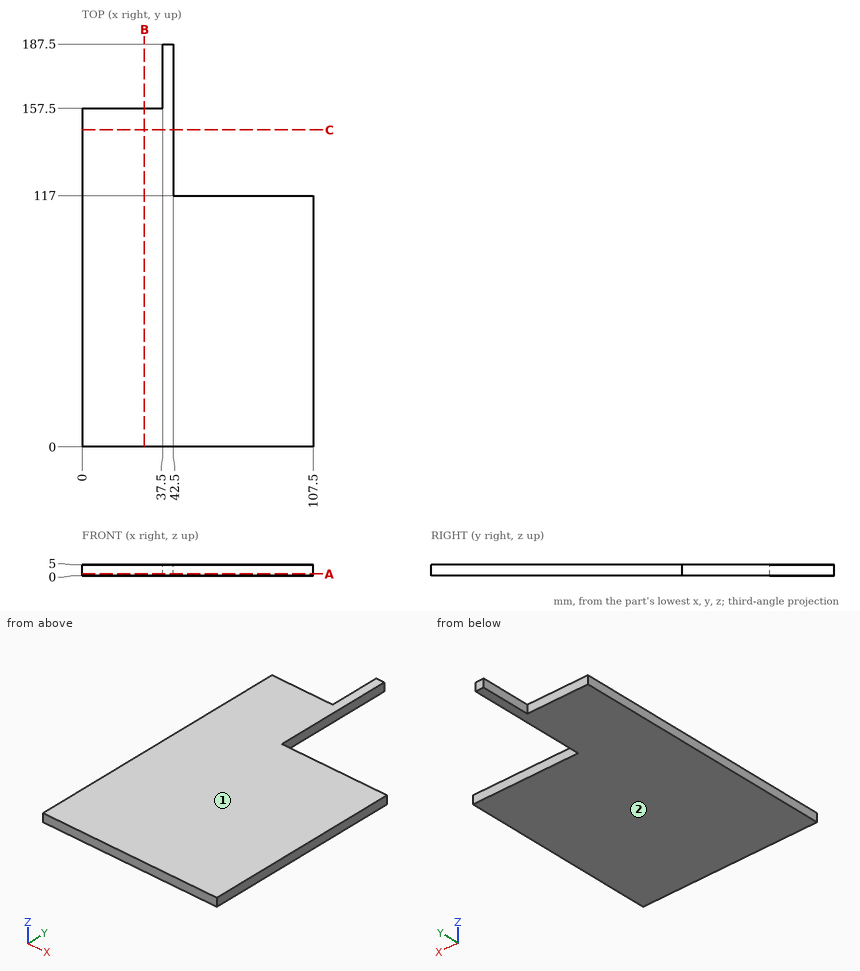
Could you check a few things on this drawing? It's one solid part, dimensions in mm from its lowest x, y, z. Coordinates: 2 decimals unless noted, no trailing zeros. Write each loop counter-clockwise with the first axis right and the second up, starting at its lowest first coordinate (ties: lowest second). Pieces come first, ordered by that corner, then holes. Notation, with made-up numbers: M 13.5,-34 L 40.5,-34 A25 ccw 40.5,-1 Z; hole C 51.25,66 d10. An arc over 180 degrees is marked long. Answer as CSV lines item,"result". Start each with the question number.
Q1. Suppose I cut it at A-A, the plane z = 0.8. List the corners of the cut face in (x, y) for me.
Q2. Suppose I cut it at C-C, the plane y = 147.5. List the corners of the cut face in (x, z) for me.
Q3. I need wall thicknesses on probe 1 along X at (y, z) = (162, 1); probe 2 along Y at (x, z) = (8.5, 4.1); probe 3 along Y at (x, z) = (48, 2.8). Which ranges of each line are inside material? Lowest first, please. Write a range as [from, to].
Q4. Will these pins go through, and if not, where does the flat tip stop? pin 1 Ø3 at (x, z) = (49.5, 1.5) entering from -Y; pin 2 Ø2 at (x, z) = (17, 1.5) entering from +Y; pin 3 Ø1.5 at (x, z) = (59.5, 2.5) entering from +Y.
Q5. If we mould it in two halves opening along Z, with no side actions, what happens to the marked faces 1 and 2? For each: pulls with the +Z half, pulls with the -Z half, needs draft (parallel to the pull), parting line crosses it, or undercut.
Q6. Suppose I cut it at B-B, the plane x = 29. List the corners of the cut face in (y, z) for me, then the cut area to 4 significant figures.
Entries:
1,outline,"M 0,0 L 107.5,0 L 107.5,117 L 42.5,117 L 42.5,187.5 L 37.5,187.5 L 37.5,157.5 L 0,157.5 Z"
2,outline,"M 0,0 L 42.5,0 L 42.5,5 L 0,5 Z"
3,probe 1,"x = [37.5, 42.5]"
3,probe 2,"y = [0, 157.5]"
3,probe 3,"y = [0, 117]"
4,pin 1,"stops at y = 0"
4,pin 2,"stops at y = 157.5"
4,pin 3,"stops at y = 117"
5,face 1,"pulls with the +Z half"
5,face 2,"pulls with the -Z half"
6,outline,"M 0,0 L 157.5,0 L 157.5,5 L 0,5 Z"
6,area,"787.5 mm²"
